from build123d import *
from OCP.BRepFilletAPI import BRepFilletAPI_MakeChamfer

# Parameters (mm, degrees)
SKETCH_1_W                          = 2.54
SKETCH_1_H                          = 2.54
EXTRUDE_1_DEPTH                     = 8.51
SKETCH_4_W                          = 0.7
SKETCH_4_H                          = 0.7
CUT_EXTRUDE_1_DEPTH                 = 8.21
CHAMFER_3_SIZE                      = 0.4
SKETCH_2_W                          = 0.5
SKETCH_2_H                          = 0.5
EXTRUDE_2_DEPTH                     = 3.15
CHAMFER_2_SIZE                      = 0.5
CHAMFER_2_SIZE2                     = 0.106278281
PATTERN_LINEAR_1_COUNT              = 4
PATTERN_LINEAR_1_PITCH              = 2.54
PATTERN_LINEAR_1_COUNT_DIR2         = 2
PATTERN_LINEAR_1_PITCH_DIR2         = 2.54
CHAMFER_3_OF_PATTERN_LINEAR_1_SIZE  = 0.4
CHAMFER_2_OF_PATTERN_LINEAR_1_SIZE  = 0.5
CHAMFER_2_OF_PATTERN_LINEAR_1_SIZE2 = 0.106278281


with BuildPart() as part:
    # Эскиз1 → Бобышка-Вытянуть1 (new body)
    with BuildSketch(Plane(origin=(0, 0, 0), x_dir=(-1, 0, 0), z_dir=(0, 1, 0))):
        Rectangle(SKETCH_1_W, SKETCH_1_H)
    extrude_1 = extrude(amount=EXTRUDE_1_DEPTH)

    # Эскиз4 → Вырез-Вытянуть1 (cut)
    with BuildSketch(Plane(origin=(0, 8.51, 0), x_dir=(1, 0, 0), z_dir=(0, 1, 0))):
        Rectangle(SKETCH_4_W, SKETCH_4_H)
    cut_extrude_1 = extrude(amount=-CUT_EXTRUDE_1_DEPTH, mode=Mode.SUBTRACT)

    # Фаска3
    chamfer_3_edges = [part.edges().sort_by_distance(p)[0] for p in [
        (-0.35, 8.51, 0),
        (0, 8.51, 0.35),
        (0.35, 8.51, 0),
        (0, 8.51, -0.35),
    ]]
    chamfer(chamfer_3_edges, length=CHAMFER_3_SIZE)

    # Эскиз2 → Бобышка-Вытянуть2 (add)
    with BuildSketch(Plane(origin=(0, 0, 0), x_dir=(-1, 0, 0), z_dir=(0, 1, 0))):
        Rectangle(SKETCH_2_W, SKETCH_2_H)
    extrude_2 = extrude(amount=-EXTRUDE_2_DEPTH)

    # Фаска2: one chamfer whose edges measure the first distance from different faces: ONE call of the kernel's chamfer builder (chamfer() names one face for all edges)
    chamfer_2_edges_1 = [part.edges().sort_by_distance(p)[0] for p in [
        (-0.25, -3.15, 0),
    ]]
    chamfer_2_side_1 = [part.faces().sort_by_distance(p)[0] for p in [
        (-0.25, -1.575, 0),
    ]]
    chamfer_2_edges_2 = [part.edges().sort_by_distance(p)[0] for p in [
        (0.25, -3.15, 0),
    ]]
    chamfer_2_side_2 = [part.faces().sort_by_distance(p)[0] for p in [
        (0.25, -1.575, 0),
    ]]
    chamfer_2 = BRepFilletAPI_MakeChamfer(part.part.solid().wrapped)
    for e in chamfer_2_edges_1:
        chamfer_2.Add(CHAMFER_2_SIZE, CHAMFER_2_SIZE2, e.wrapped, chamfer_2_side_1[0].wrapped)  # the first distance lies on this face
    for e in chamfer_2_edges_2:
        chamfer_2.Add(CHAMFER_2_SIZE, CHAMFER_2_SIZE2, e.wrapped, chamfer_2_side_2[0].wrapped)  # the first distance lies on this face
    add(Compound.cast(chamfer_2.Shape()), mode=Mode.REPLACE)

    # Линейный массив1: Бобышка-Вытянуть1, Вырез-Вытянуть1, Extrude 2 4 × 2
    with Locations(*[(-j * PATTERN_LINEAR_1_PITCH_DIR2, 0, -i * PATTERN_LINEAR_1_PITCH) for i in range(PATTERN_LINEAR_1_COUNT) for j in range(PATTERN_LINEAR_1_COUNT_DIR2) if (i, j) != (0, 0)]):
        add(extrude_1)
        add(cut_extrude_1, mode=Mode.SUBTRACT)
        add(extrude_2)

    # Фаска3 of Линейный массив1
    chamfer_3_of_pattern_linear_1_edges = [part.edges().sort_by_distance(p)[0] for p in [
        (-2.89, 8.51, 0),
        (-2.54, 8.51, 0.35),
        (-2.19, 8.51, 0),
        (-2.54, 8.51, -0.35),
        (-0.35, 8.51, -2.54),
        (0, 8.51, -2.19),
        (0.35, 8.51, -2.54),
        (0, 8.51, -2.89),
        (-2.89, 8.51, -2.54),
        (-2.54, 8.51, -2.19),
        (-2.19, 8.51, -2.54),
        (-2.54, 8.51, -2.89),
        (-0.35, 8.51, -5.08),
        (0, 8.51, -4.73),
        (0.35, 8.51, -5.08),
        (0, 8.51, -5.43),
        (-2.89, 8.51, -5.08),
        (-2.54, 8.51, -4.73),
        (-2.19, 8.51, -5.08),
        (-2.54, 8.51, -5.43),
        (-0.35, 8.51, -7.62),
        (0, 8.51, -7.27),
        (0.35, 8.51, -7.62),
        (0, 8.51, -7.97),
        (-2.89, 8.51, -7.62),
        (-2.54, 8.51, -7.27),
        (-2.19, 8.51, -7.62),
        (-2.54, 8.51, -7.97),
    ]]
    chamfer(chamfer_3_of_pattern_linear_1_edges, length=CHAMFER_3_OF_PATTERN_LINEAR_1_SIZE)

    # Фаска2 of Линейный массив1: one chamfer whose edges measure the first distance from different faces: ONE call of the kernel's chamfer builder (chamfer() names one face for all edges)
    chamfer_2_of_pattern_linear_1_edges_1 = [part.edges().sort_by_distance(p)[0] for p in [
        (-2.79, -3.15, 0),
    ]]
    chamfer_2_of_pattern_linear_1_side_1 = [part.faces().sort_by_distance(p)[0] for p in [
        (-2.79, -1.575, 0),
    ]]
    chamfer_2_of_pattern_linear_1_edges_2 = [part.edges().sort_by_distance(p)[0] for p in [
        (-2.29, -3.15, 0),
    ]]
    chamfer_2_of_pattern_linear_1_side_2 = [part.faces().sort_by_distance(p)[0] for p in [
        (-2.29, -1.575, 0),
    ]]
    chamfer_2_of_pattern_linear_1_edges_3 = [part.edges().sort_by_distance(p)[0] for p in [
        (-0.25, -3.15, -2.54),
    ]]
    chamfer_2_of_pattern_linear_1_side_3 = [part.faces().sort_by_distance(p)[0] for p in [
        (-0.25, -1.575, -2.54),
    ]]
    chamfer_2_of_pattern_linear_1_edges_4 = [part.edges().sort_by_distance(p)[0] for p in [
        (0.25, -3.15, -2.54),
    ]]
    chamfer_2_of_pattern_linear_1_side_4 = [part.faces().sort_by_distance(p)[0] for p in [
        (0.25, -1.575, -2.54),
    ]]
    chamfer_2_of_pattern_linear_1_edges_5 = [part.edges().sort_by_distance(p)[0] for p in [
        (-2.79, -3.15, -2.54),
    ]]
    chamfer_2_of_pattern_linear_1_side_5 = [part.faces().sort_by_distance(p)[0] for p in [
        (-2.79, -1.575, -2.54),
    ]]
    chamfer_2_of_pattern_linear_1_edges_6 = [part.edges().sort_by_distance(p)[0] for p in [
        (-2.29, -3.15, -2.54),
    ]]
    chamfer_2_of_pattern_linear_1_side_6 = [part.faces().sort_by_distance(p)[0] for p in [
        (-2.29, -1.575, -2.54),
    ]]
    chamfer_2_of_pattern_linear_1_edges_7 = [part.edges().sort_by_distance(p)[0] for p in [
        (-0.25, -3.15, -5.08),
    ]]
    chamfer_2_of_pattern_linear_1_side_7 = [part.faces().sort_by_distance(p)[0] for p in [
        (-0.25, -1.575, -5.08),
    ]]
    chamfer_2_of_pattern_linear_1_edges_8 = [part.edges().sort_by_distance(p)[0] for p in [
        (0.25, -3.15, -5.08),
    ]]
    chamfer_2_of_pattern_linear_1_side_8 = [part.faces().sort_by_distance(p)[0] for p in [
        (0.25, -1.575, -5.08),
    ]]
    chamfer_2_of_pattern_linear_1_edges_9 = [part.edges().sort_by_distance(p)[0] for p in [
        (-2.79, -3.15, -5.08),
    ]]
    chamfer_2_of_pattern_linear_1_side_9 = [part.faces().sort_by_distance(p)[0] for p in [
        (-2.79, -1.575, -5.08),
    ]]
    chamfer_2_of_pattern_linear_1_edges_10 = [part.edges().sort_by_distance(p)[0] for p in [
        (-2.29, -3.15, -5.08),
    ]]
    chamfer_2_of_pattern_linear_1_side_10 = [part.faces().sort_by_distance(p)[0] for p in [
        (-2.29, -1.575, -5.08),
    ]]
    chamfer_2_of_pattern_linear_1_edges_11 = [part.edges().sort_by_distance(p)[0] for p in [
        (-0.25, -3.15, -7.62),
    ]]
    chamfer_2_of_pattern_linear_1_side_11 = [part.faces().sort_by_distance(p)[0] for p in [
        (-0.25, -1.575, -7.62),
    ]]
    chamfer_2_of_pattern_linear_1_edges_12 = [part.edges().sort_by_distance(p)[0] for p in [
        (0.25, -3.15, -7.62),
    ]]
    chamfer_2_of_pattern_linear_1_side_12 = [part.faces().sort_by_distance(p)[0] for p in [
        (0.25, -1.575, -7.62),
    ]]
    chamfer_2_of_pattern_linear_1_edges_13 = [part.edges().sort_by_distance(p)[0] for p in [
        (-2.79, -3.15, -7.62),
    ]]
    chamfer_2_of_pattern_linear_1_side_13 = [part.faces().sort_by_distance(p)[0] for p in [
        (-2.79, -1.575, -7.62),
    ]]
    chamfer_2_of_pattern_linear_1_edges_14 = [part.edges().sort_by_distance(p)[0] for p in [
        (-2.29, -3.15, -7.62),
    ]]
    chamfer_2_of_pattern_linear_1_side_14 = [part.faces().sort_by_distance(p)[0] for p in [
        (-2.29, -1.575, -7.62),
    ]]
    chamfer_2_of_pattern_linear_1 = BRepFilletAPI_MakeChamfer(part.part.solid().wrapped)
    for e in chamfer_2_of_pattern_linear_1_edges_1:
        chamfer_2_of_pattern_linear_1.Add(CHAMFER_2_OF_PATTERN_LINEAR_1_SIZE, CHAMFER_2_OF_PATTERN_LINEAR_1_SIZE2, e.wrapped, chamfer_2_of_pattern_linear_1_side_1[0].wrapped)  # the first distance lies on this face
    for e in chamfer_2_of_pattern_linear_1_edges_2:
        chamfer_2_of_pattern_linear_1.Add(CHAMFER_2_OF_PATTERN_LINEAR_1_SIZE, CHAMFER_2_OF_PATTERN_LINEAR_1_SIZE2, e.wrapped, chamfer_2_of_pattern_linear_1_side_2[0].wrapped)  # the first distance lies on this face
    for e in chamfer_2_of_pattern_linear_1_edges_3:
        chamfer_2_of_pattern_linear_1.Add(CHAMFER_2_OF_PATTERN_LINEAR_1_SIZE, CHAMFER_2_OF_PATTERN_LINEAR_1_SIZE2, e.wrapped, chamfer_2_of_pattern_linear_1_side_3[0].wrapped)  # the first distance lies on this face
    for e in chamfer_2_of_pattern_linear_1_edges_4:
        chamfer_2_of_pattern_linear_1.Add(CHAMFER_2_OF_PATTERN_LINEAR_1_SIZE, CHAMFER_2_OF_PATTERN_LINEAR_1_SIZE2, e.wrapped, chamfer_2_of_pattern_linear_1_side_4[0].wrapped)  # the first distance lies on this face
    for e in chamfer_2_of_pattern_linear_1_edges_5:
        chamfer_2_of_pattern_linear_1.Add(CHAMFER_2_OF_PATTERN_LINEAR_1_SIZE, CHAMFER_2_OF_PATTERN_LINEAR_1_SIZE2, e.wrapped, chamfer_2_of_pattern_linear_1_side_5[0].wrapped)  # the first distance lies on this face
    for e in chamfer_2_of_pattern_linear_1_edges_6:
        chamfer_2_of_pattern_linear_1.Add(CHAMFER_2_OF_PATTERN_LINEAR_1_SIZE, CHAMFER_2_OF_PATTERN_LINEAR_1_SIZE2, e.wrapped, chamfer_2_of_pattern_linear_1_side_6[0].wrapped)  # the first distance lies on this face
    for e in chamfer_2_of_pattern_linear_1_edges_7:
        chamfer_2_of_pattern_linear_1.Add(CHAMFER_2_OF_PATTERN_LINEAR_1_SIZE, CHAMFER_2_OF_PATTERN_LINEAR_1_SIZE2, e.wrapped, chamfer_2_of_pattern_linear_1_side_7[0].wrapped)  # the first distance lies on this face
    for e in chamfer_2_of_pattern_linear_1_edges_8:
        chamfer_2_of_pattern_linear_1.Add(CHAMFER_2_OF_PATTERN_LINEAR_1_SIZE, CHAMFER_2_OF_PATTERN_LINEAR_1_SIZE2, e.wrapped, chamfer_2_of_pattern_linear_1_side_8[0].wrapped)  # the first distance lies on this face
    for e in chamfer_2_of_pattern_linear_1_edges_9:
        chamfer_2_of_pattern_linear_1.Add(CHAMFER_2_OF_PATTERN_LINEAR_1_SIZE, CHAMFER_2_OF_PATTERN_LINEAR_1_SIZE2, e.wrapped, chamfer_2_of_pattern_linear_1_side_9[0].wrapped)  # the first distance lies on this face
    for e in chamfer_2_of_pattern_linear_1_edges_10:
        chamfer_2_of_pattern_linear_1.Add(CHAMFER_2_OF_PATTERN_LINEAR_1_SIZE, CHAMFER_2_OF_PATTERN_LINEAR_1_SIZE2, e.wrapped, chamfer_2_of_pattern_linear_1_side_10[0].wrapped)  # the first distance lies on this face
    for e in chamfer_2_of_pattern_linear_1_edges_11:
        chamfer_2_of_pattern_linear_1.Add(CHAMFER_2_OF_PATTERN_LINEAR_1_SIZE, CHAMFER_2_OF_PATTERN_LINEAR_1_SIZE2, e.wrapped, chamfer_2_of_pattern_linear_1_side_11[0].wrapped)  # the first distance lies on this face
    for e in chamfer_2_of_pattern_linear_1_edges_12:
        chamfer_2_of_pattern_linear_1.Add(CHAMFER_2_OF_PATTERN_LINEAR_1_SIZE, CHAMFER_2_OF_PATTERN_LINEAR_1_SIZE2, e.wrapped, chamfer_2_of_pattern_linear_1_side_12[0].wrapped)  # the first distance lies on this face
    for e in chamfer_2_of_pattern_linear_1_edges_13:
        chamfer_2_of_pattern_linear_1.Add(CHAMFER_2_OF_PATTERN_LINEAR_1_SIZE, CHAMFER_2_OF_PATTERN_LINEAR_1_SIZE2, e.wrapped, chamfer_2_of_pattern_linear_1_side_13[0].wrapped)  # the first distance lies on this face
    for e in chamfer_2_of_pattern_linear_1_edges_14:
        chamfer_2_of_pattern_linear_1.Add(CHAMFER_2_OF_PATTERN_LINEAR_1_SIZE, CHAMFER_2_OF_PATTERN_LINEAR_1_SIZE2, e.wrapped, chamfer_2_of_pattern_linear_1_side_14[0].wrapped)  # the first distance lies on this face
    add(Compound.cast(chamfer_2_of_pattern_linear_1.Shape()), mode=Mode.REPLACE)


solid = part.part
Build history of the part. All positions in model axes, mm. Give positions to 0.01 mm unless a question says otherwise; leave off trailing zeros. Order: outer loops, then holes, each group sorted by start corner. A loop starts at its lowest first (then second) coordinate and runs counter-clockwise, first axis right, second up. Notation, with made-up numbers: M -18.75,-12.75 L -12.75,-12.75 A14 cw -12.75,13.25 Z; hole C 47.5,39.5 d9. An arc over 180 degrees is marked long. Put each result on its own line as item: value.
Item 1: Probe line 1 (X direction, y = 2, z = -2.75); line 2 (Z direction, x = 0.2, y = -2); line 3 (Z direction, x = 0.1, y = 7.5). List the from-to ranges inside material, lowest first. Write a range as [from, to].
From the geometry:
line 1: x = [-3.81, -2.89], [-2.19, -0.35], [0.35, 1.27]
line 2: z = [-7.87, -7.37], [-5.33, -4.83], [-2.79, -2.29], [-0.25, 0.25]
line 3: z = [-8.89, -7.97], [-7.27, -5.43], [-4.73, -2.89], [-2.19, -0.35], [0.35, 1.27]
Item 2: Two-plate mould, pull along Z, no slides. Class faces 1 (the flat face through (-3.81, 4, -4)), 2 (the flat face through (-1, 0, -4)), 3 (the flat face through (-1, 4, -8.89)): +Z half, -Z half, draft (parallel to the pull), parting line (faces both ways), or undercut.
From the geometry:
face 1: draft
face 2: undercut
face 3: -Z half
Item 3: Slice it at A-A, the plane z = -0.5. Write the cut outline in (x, y), plus the area to 3 significant figures.
From the geometry:
outline: M -3.81,0 L 1.27,0 L 1.27,8.51 L 0.75,8.51 L 0.5,8.26 L -0.5,8.26 L -0.75,8.51 L -1.79,8.51 L -2.04,8.26 L -3.04,8.26 L -3.29,8.51 L -3.81,8.51 Z
area: 42.6 mm2
Item 4: Slice it at B-B, the plane y = 5.25. Give the number of separate pieces and of enclosed holes in the cut face, plus the area to 3 significant figures.
From the geometry:
separate pieces: 1
enclosed holes: 8
area: 47.7 mm2
Item 5: Slice it at C-C, the plane x = -3.5. Write the cut outline in (y, z).
From the geometry:
outline: M 0,-8.89 L 8.51,-8.89 L 8.51,1.27 L 0,1.27 Z
Item 6: Flat gauge pins, fed straight in: pin 1 Ø0.6 at (x, y) = (0, -1.5) entering from +Z; pin 2 Ø0.6 at (x, y) = (-2.5, -1) entering from -Z. Where does each tip first touch, or does it go through?
From the geometry:
pin 1: stops at z = 0.25
pin 2: stops at z = -7.87
